Part model, mm, in its own coordinate system. Face numbers are marked on the shaded views. A direction names the side the tool comes from. Give positions to 0.01 mm unless a question says otherwise; leave off trailing zeros. Loops run counter-clockwise (first coordinate to the right, second up) from the corner with the lowest first, then second, coordinate; pieces in that order, holes last. Notation, with made-up numbers: (-30, 57.25) -> (-14, 57.25) arc R20 cw to (-14, 86.25) -> close; hole circle Ø3 at (89.5, -5). An arc over 180 degrees is marked (long way). Write item = value, one per line.
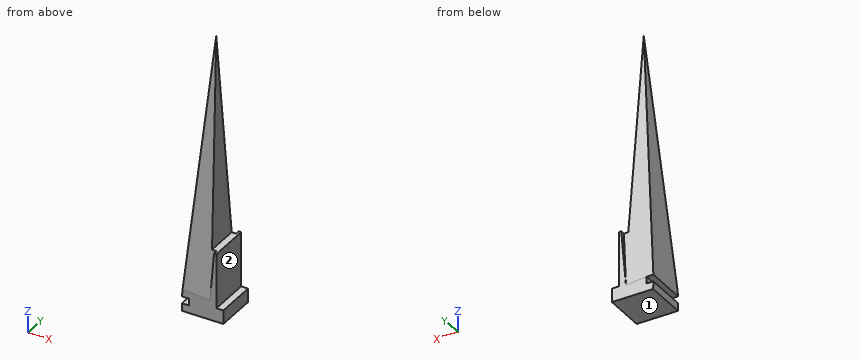
from build123d import *

# Parameters (mm, degrees)
F1_DEPTH = 76.2
F4_DEPTH = 25.4
F6_DEPTH = 25.4
F7_DEPTH = 25.4
F8_DEPTH = 25.4


with BuildPart() as f1:
    # F0 (on Front) → F1 (new body)
    with BuildSketch(Plane.XZ):
        Polygon((-40.0857904882, 1.7159489595), (36.1142095118, 1.7159489595), (36.1142095118, 27.1159489595), (23.4142095118, 27.1159489595), (23.4142095118, 128.7159489595), (10.7142095118, 128.7159489595), (0, 509.5652704956), (-40.4825732112, 28.6661945283), (-27.7825732112, 28.6661945283), (-27.7825732112, 15.9661945283), (-40.4825732112, 15.9661945283), align=None)
    extrude(amount=F1_DEPTH)

    # F3 (on face) → F4 (cut)
    with BuildSketch(Plane(origin=(-42.5938834628, 0, 3.585596421), x_dir=(0, -1, 0), z_dir=(-0.9964754993, 0, 0.0838843208))):
        Polygon((37.7841320195, 507.7693073485), (76.2, 38.4734290846), (76.2, 507.7693073485), align=None)
    extrude(amount=-F4_DEPTH, mode=Mode.SUBTRACT)

    # F5 (on face) → F6 (cut)
    with BuildSketch(Plane(origin=(-42.5938834628, 0, 3.585596421), x_dir=(0, -1, 0), z_dir=(-0.9964754993, 0, 0.0838843208))):
        Polygon((0, 25.9728506207), (37.9639834193, 507.7693073485), (0, 507.7693073485), align=None)
    extrude(amount=-F6_DEPTH, mode=Mode.SUBTRACT)

    # F7 (cut): a face of the model
    f7_faces = [f1.faces().sort_by_distance(p)[0] for p in [
        (-0.4288778428, -69.5509425431, 201.6726152219),
    ]]
    extrude(f7_faces, amount=-F7_DEPTH, mode=Mode.SUBTRACT)

    # F8 (cut): a face of the model
    f8_faces = [f1.faces().sort_by_distance(p)[0] for p in [
        (-0.7784120208, -6.7286940969, 197.5204418331),
    ]]
    extrude(f8_faces, amount=-F8_DEPTH, mode=Mode.SUBTRACT)


solid = f1.part
1) Drop flat-ended pins along their axis: P1, Ø5, axis at x = 6.5, z = 162.5, coming from the +Y side; P2, Ø1.5, axis at x = 13, z = 100, coming from the -Y side; P3, Ø4, axis at y = -17.5, z = 273, coming from the +X side; P4, Ø8, axis at x = 13, z = 234, coming from the -Y side (3 decimals). Give the stop position or say it passes through.
Resolved:
P1 = -10.56
P2 = -71.16
P3 = 6.67
P4 = through
2) Slice it at A-A, the plane y = -47.5. List the corners of the cut face in (x, z).
Resolved:
outline = (-40.48, 15.97) -> (-40.09, 1.72) -> (36.11, 1.72) -> (36.11, 27.12) -> (23.41, 27.12) -> (23.41, 128.72) -> (10.71, 128.72) -> (3.36, 390.17) -> (-9.96, 391.29) -> (-40.48, 28.67) -> (-27.78, 28.67) -> (-27.78, 15.97) -> close
3) Slice it at B-B, the plane x = 31. List the corners of the cut face in (y, z).
Resolved:
outline = (-76.2, 1.72) -> (0, 1.72) -> (0, 27.12) -> (-76.2, 27.12) -> close
4) Slice it at C-C, the plane z = 84. List the corners of the cut face in (x, y), and give its area (3 significant figures).
Resolved:
outline = (-35.82, -72.74) -> (15.16, -72.39) -> (15.16, -76.2) -> (23.41, -76.2) -> (23.41, 0) -> (15.16, 0) -> (15.16, -4.65) -> (-35.82, -4.31) -> close
area = 4,100 mm²
5) Slice it at D-D, the plane y = -17.5. List the corners of the cut face in (x, z), and give its area (3 significant figures).
Resolved:
outline = (-40.48, 15.97) -> (-40.09, 1.72) -> (36.11, 1.72) -> (36.11, 27.12) -> (23.41, 27.12) -> (23.41, 128.72) -> (10.71, 128.72) -> (7.35, 248.32) -> (-21.79, 250.77) -> (-40.48, 28.67) -> (-27.78, 28.67) -> (-27.78, 15.97) -> close
area = 12,200 mm²
6) Which spindle directions (+Z, -Z, +X, -X, +Y, -Y) get a long thin tool onto all of the face, cutting with end or side? Do the marked faces 1 and 2. Say none if no direction does.
Resolved:
face_1 = -Z, +X, -X, +Y, -Y
face_2 = +Z, +X, +Y, -Y
7) Drill centre lines: line 1 along Z through (x, y) = (14, -59); line 2 along X through (y, z) = (-30, 317); line 3 along Y through (x, z) = (-35.5, 45.5). Where is each one in solid material? Low to high. Write a range as [from, to].
Resolved:
line_1 = [1.72, 128.72]
line_2 = [-16.21, 5.42]
line_3 = [-75.88, -1.29]
